from build123d import *

# Parameters (mm, degrees)
SKETCH1_R           = 3
SKETCH1_R_2         = 5
BOSS_EXTRUDE2_DEPTH = 7.5
BOSS_EXTRUDE3_DEPTH = 6.5
FILLET1_R           = 3


with BuildPart() as part:
    # Sketch1 → Boss-Extrude2 (new body, symmetric)
    with BuildSketch(Plane.XY):
        with BuildLine():
            Line((95.02071112, 4.178119463), (3.897114317, 2.25))
            ThreePointArc((3.897114317, 2.25), (-4.5, 0), (3.897114317, -2.25))
            Line((3.897114317, -2.25), (95.02071112, -4.178119463))
            ThreePointArc((95.02071112, -4.178119463), (106.5, 0), (95.02071112, 4.178119463))
        make_face()
        with BuildLine():
            ThreePointArc((7.883680433, -1.059645666), (6.824034767, 0), (7.883680433, 1.059645666))
            Line((7.883680433, 1.059645666), (88.855952705, 2.772969323))
            ThreePointArc((88.855952705, 2.772969323), (91.748807392, 0), (88.855952705, -2.772969323))
            Line((88.855952705, -2.772969323), (7.883680433, -1.059645666))
        make_face(mode=Mode.SUBTRACT)
        Circle(SKETCH1_R, mode=Mode.SUBTRACT)
        with Locations((100, 0)):
            Circle(SKETCH1_R_2, mode=Mode.SUBTRACT)
    extrude(amount=BOSS_EXTRUDE2_DEPTH, both=True)

    # Sketch1_7 → Boss-Extrude3 (add, symmetric)
    with BuildSketch(Plane.XY):
        with BuildLine():
            Line((88.855952705, 2.772969323), (7.883680433, 1.059645666))
            ThreePointArc((7.883680433, 1.059645666), (6.824034767, 0), (7.883680433, -1.059645666))
            Line((7.883680433, -1.059645666), (88.855952705, -2.772969323))
            Line((88.855952705, -2.772969323), (88.973353931, -2.775453461))
            ThreePointArc((88.973353931, -2.775453461), (91.748807392, 0), (88.973353931, 2.775453461))
            Line((88.973353931, 2.775453461), (88.855952705, 2.772969323))
        make_face()
    extrude(amount=BOSS_EXTRUDE3_DEPTH, both=True)

    # Fillet1
    fillet1_edges = [part.edges().sort_by_distance(p)[0] for p in [
        (3.897114317, -2.25, 0),
        (3.897114317, 2.25, 0),
        (95.02071112, 4.178119463, 0),
        (95.02071112, -4.178119463, 0),
    ]]
    fillet(fillet1_edges, radius=FILLET1_R)


solid = part.part
Source: CAD feature listing. Evaluate the final solid. Frame: model axes, mm. A direction names the side the tool comes from. Round coordinates to 2 decimals unless told otherwise and drop trailing zeros. Loops run counter-clockwise (first coordinate to the right, second up) from the corner with the lowest first, then second, coordinate; pieces in that order, holes last. Notation, with made-up numbers: (64, -7.75) -> (81, -7.75) arc R24 cw to (81, 6.25) -> close; hole circle Ø2 at (57, 71.5). An arc over 180 degrees is marked (long way). Answer as a JSON object with one key per item and string values. Group by question number.
Q1. Mould query, pull axis Y, two halves, no side actions, for faces 1 (the cylindrical face through (-3, 0, 0)), 2 (the cylindrical face through (4.2, -2.5, 0.1)), 3 (the cylindrical face through (4.2, 2.5, 0.1)), 4 (the flat face through (55, 3, -7.5)). Classes: pulls with the +Y half, pulls with the -Y half, needs draft (parallel to the pull), parting line crosses it, or undercut.
Q2. Section query D-D (x = 55). Output: boundary loops of the cut face in (y, z).
Q3. Section query C-C (y = 0). Output: boundary loops of the cut face in (x, z).
Q4. Ray query, line 1 (Y direction, x = 0, z = 3); line 2 (Y direction, x = 100, z = 4.5); line 3 (Z direction, x = 60, y = 2). Return the intervals inside material, ascending. Write a range as from..to.
Q5. Access query for faces 5 (the flat face through (58, 0, 6.5)), 6 (the flat face through (58, 0, -6.5)), 7 (the cylindrical face through (94.84, -4.36, -0.11)). Directions: +Z, -Z, +X, -X, +Y, -Y. A direction counts if a zero-diameter tool reaches every point of the face in a straight line with its end or side. Return the directions, or none.
Q6. Section query B-B (x = 100). Output: boundary loops of the cut face in (y, z).
Q7. Contact query for flat-ended pins moving along their axis: P1, Ø1, axis at x = 51, z = 5.5, coming from the -Y side; P2, Ø1.5, axis at x = 40.5, z = 3.5, coming from the -Y side; P3, Ø5, axis at x = 25.5, z = 5.5, coming from the +Y side. Output: stop coordinate, or through.
Completed:
{
 "1": {"face 1": "undercut", "face 2": "pulls with the -Y half", "face 3": "pulls with the +Y half", "face 4": "needs draft"},
 "2": {"outline": "(-3.33, -7.5) -> (-2.06, -7.5) -> (-2.06, -6.5) -> (2.06, -6.5) -> (2.06, -7.5) -> (3.33, -7.5) -> (3.33, 7.5) -> (2.06, 7.5) -> (2.06, 6.5) -> (-2.06, 6.5) -> (-2.06, 7.5) -> (-3.33, 7.5) -> close"},
 "3": {"outline": "(-4.5, -7.5) -> (-3, -7.5) -> (-3, 7.5) -> (-4.5, 7.5) -> close; (3, -7.5) -> (6.82, -7.5) -> (6.82, -6.5) -> (91.75, -6.5) -> (91.75, -7.5) -> (95, -7.5) -> (95, 7.5) -> (91.75, 7.5) -> (91.75, 6.5) -> (6.82, 6.5) -> (6.82, 7.5) -> (3, 7.5) -> close; (105, -7.5) -> (106.5, -7.5) -> (106.5, 7.5) -> (105, 7.5) -> close"},
 "4": {"line 1": "-4.5..-3, 3..4.5", "line 2": "-6.5..-5, 5..6.5", "line 3": "-6.5..6.5"},
 "5": {"face 5": "+Z", "face 6": "-Z", "face 7": "+Z, -Z, -Y"},
 "6": {"outline": "(-6.5, -7.5) -> (-5, -7.5) -> (-5, 7.5) -> (-6.5, 7.5) -> close; (5, -7.5) -> (6.5, -7.5) -> (6.5, 7.5) -> (5, 7.5) -> close"},
 "7": {"P1": "y = -3.26", "P2": "y = -3.04", "P3": "y = 2.76"}
}
